```python
from build123d import *

# Parameters (mm, degrees)
ESTRUSIONE_ESTRUSIONE1_DEPTH                         = 4
ESTRUSIONE_ESTRUSIONE2_START                         = -36
ESTRUSIONE_ESTRUSIONE2_DEPTH                         = 36
ESTRUSIONE_ESTRUSIONE3_START                         = -46
ESTRUSIONE_ESTRUSIONE3_DEPTH                         = 46
SMUSSO3_SIZE                                         = 8.0941
SMUSSO3_SIZE2                                        = 11.999996735
SMUSSO2_SIZE                                         = 8.0941
SMUSSO2_SIZE_2                                       = 11.999996735
FORO_LAMATO_PER_VITE_M4_A_TESTA_CILINDRI_D           = 4.5
FORO_LAMATO_PER_VITE_M4_A_TESTA_CILINDRI_DEPTH       = 50
FORO_LAMATO_PER_VITE_M4_A_TESTA_CILINDRI_CBORE_D     = 8
FORO_LAMATO_PER_VITE_M4_A_TESTA_CILINDRI_CBORE_DEPTH = 35.6
FORO_LAMATO_PER_VITE_M4_A_TESTA_CILINDRI_TIP         = 1.351936393
FORO_PER_VITE_M4_1_D                                 = 4.5
FORO_PER_VITE_M4_1_DEPTH                             = 50
FORO_PER_VITE_M4_1_TIP                               = 1.351936393


with BuildPart() as part:
    # Schizzo1 → Estrusione-Estrusione1 (new body)
    with BuildSketch(Plane.XY):
        Polygon((35, 30), (23, 30), (23, 18), (23, 0), (-23, 0), (-23, 18), (-23, 30), (-35, 30), (-35, -12), (35, -12), align=None)
        with BuildLine():
            ThreePointArc((-8, 18), (0, 10), (8, 18))
            Line((8, 18), (23, 18))
            Line((23, 18), (23, 0))
            Line((23, 0), (-23, 0))
            Line((-23, 0), (-23, 18))
            Line((-23, 18), (-8, 18))
        make_face()
    extrude(amount=ESTRUSIONE_ESTRUSIONE1_DEPTH)

    # Schizzo1<3> → Estrusione-Estrusione2 (add)
    with BuildSketch(Plane.XY.offset(ESTRUSIONE_ESTRUSIONE2_START)):
        with BuildLine():
            ThreePointArc((-8, 18), (0, 10), (8, 18))
            Line((8, 18), (23, 18))
            Line((23, 18), (23, 0))
            Line((23, 0), (-23, 0))
            Line((-23, 0), (-23, 18))
            Line((-23, 18), (-8, 18))
        make_face()
    extrude(amount=ESTRUSIONE_ESTRUSIONE2_DEPTH)

    # Schizzo6 → Estrusione-Estrusione3 (add)
    with BuildSketch(Plane(origin=(23, 0, 0), x_dir=(0, 0, -1), z_dir=(1, 0, 0)).offset(ESTRUSIONE_ESTRUSIONE3_START)):
        Polygon((0, 0), (25, 0), (0, -12), align=None)
    extrude(amount=ESTRUSIONE_ESTRUSIONE3_DEPTH)

    # Smusso3
    smusso3_edges = [part.edges().sort_by_distance(p)[0] for p in [
        (-23, 3, 0),
    ]]
    smusso3_side = [part.faces().sort_by_distance(p)[0] for p in [
        (-23, 6.556390977, -16.182957393),
    ]]
    chamfer(smusso3_edges, length=SMUSSO3_SIZE, length2=SMUSSO3_SIZE2, reference=smusso3_side[0])

    # Smusso2
    # the kernel refuses this chamfer: 11.999996735, 8.0941 mm, written as the material it adds along each edge
    with BuildSketch(Plane(origin=(23, -43.002099643, 0), x_dir=(-0.047532142988028575, 0, -0.9988697089125115), z_dir=(0, 1, 0))) as smusso2_piece_1_section:
        Polygon((SMUSSO2_SIZE * 0.998869708913, -SMUSSO2_SIZE * 0.047532142988), (-SMUSSO2_SIZE_2 * 0.047532142989, -SMUSSO2_SIZE_2 * 0.998869708932), (0, 0), align=None)
    smusso2_piece_1 = extrude(amount=61.002099643, mode=Mode.PRIVATE)
    smusso2_piece_1 = split(smusso2_piece_1, bisect_by=Plane(origin=(27.04511503, -8.043833676, -8.242013176), z_dir=(0, 0.9015230574682735, 0.4327310675847713)), keep=Keep.TOP, mode=Mode.PRIVATE)
    add(smusso2_piece_1)

    # Foro lamato per Vite M4 a testa cilindrica piana-1
    with Locations(Plane(origin=(0, 0, -36), x_dir=(-1, 0, 0), z_dir=(0, 0, -1))):
        with Locations((-29, -6), (28.999998368, -6)):
            CounterBoreHole(FORO_LAMATO_PER_VITE_M4_A_TESTA_CILINDRI_D / 2, FORO_LAMATO_PER_VITE_M4_A_TESTA_CILINDRI_CBORE_D / 2, FORO_LAMATO_PER_VITE_M4_A_TESTA_CILINDRI_CBORE_DEPTH, depth=FORO_LAMATO_PER_VITE_M4_A_TESTA_CILINDRI_DEPTH)
            with Locations((0, 0, -(FORO_LAMATO_PER_VITE_M4_A_TESTA_CILINDRI_DEPTH + FORO_LAMATO_PER_VITE_M4_A_TESTA_CILINDRI_TIP / 2))):  # 118° drill point
                Cone(0, FORO_LAMATO_PER_VITE_M4_A_TESTA_CILINDRI_D / 2, FORO_LAMATO_PER_VITE_M4_A_TESTA_CILINDRI_TIP, mode=Mode.SUBTRACT)

    # Foro per Vite M4-1
    with Locations(Plane(origin=(29, 24, 0), x_dir=(-1, 0, 0), z_dir=(0, 0, -1))):
        with Locations((0, 0), (58, 0)):
            Hole(FORO_PER_VITE_M4_1_D / 2, depth=FORO_PER_VITE_M4_1_DEPTH)
            with Locations((0, 0, -(FORO_PER_VITE_M4_1_DEPTH + FORO_PER_VITE_M4_1_TIP / 2))):  # 118° drill point
                Cone(0, FORO_PER_VITE_M4_1_D / 2, FORO_PER_VITE_M4_1_TIP, mode=Mode.SUBTRACT)


solid = part.part
```
Geometry check sheet. Reference: the model listing, model coordinates, mm. A direction names the side the tool comes from. Coordinates: 2 decimals unless noted, no trailing zeros. Order: outer loops, then holes, each group sorted by start corner. A loop starts at its lowest first (then second) coordinate and runs counter-clockwise, first axis right, second up. Notation, with made-up numbers: (39, 26.5) - (87, 26.5) arc R24 cw to (87, 48.5) - close; hole circle Ø8 at (58, 34). An arc over 180 degrees is marked (long way). Answer in a Markdown table with one row per item. Add a question column.
1. Material ranges on L1, parallel to Y at x = 29, z = 2.5; L2, parallel to X at y = -0.5, z = -20; L3, parallel to X at y = -6, z = -3, recorded low to high. Write a range as [from, to].
2. Section check B-B (y = 19). Enter the section's corners in (x, z), plus the area to 3 significant figures.
3. Section check C-C (z = -15). Enter the section's corners in (x, y).
4. Gauge pin test, flat ends, axial feed: pin 1 Ø8 at (x, z) = (-16.5, -25.5) entering from +Y; pin 2 Ø8 at (y, z) = (-5.5, -23) entering from -X; pin 3 Ø8 at (y, z) = (-0.5, -18.5) entering from -X; pin 4 Ø7 at (x, y) = (29, -6) entering from -Z. Record the tip position at first contact, or that the pin passes through.
5. Draft check along X on faces 1 (the face through (0, 9, -36)), 2 (the face through (28.92, 6.12, -4.1)), 3 (the face through (23, 24, 2)), 4 (the face through (-23, 24, 2)). Enter one of: +X half, -X half, draft (parallel to the pull), parting line (faces both ways), or undercut.
6. Access from +Z, -Z, +X, -X, +Y, -Y to the whole of each face (thin tool, end or side, straight path). Record for faces 5 (the face through (23, 8, -22)), 6 (the face through (29, 21.5, 0)), 7 (the face through (0, 0, -31)), 8 (the face through (-23, 8, -22)).
7. Section check A-A (y = 24). Enter the section's corners in (x, z).
Data:
| question | item | result |
|---|---|---|
| 1 | L1 | y = [-12, -8.25], [-3.75, 21.75], [26.25, 30] |
| 1 | L2 | x = [-23, 23] |
| 1 | L3 | x = [-25, 25] |
| 2 | outline | (-35, 0) - (-23, 0) - (-23, 4) - (-35, 4) - close; (23, 0) - (35, 0) - (35, 4) - (23, 4) - close |
| 2 | area | 96.0 mm² |
| 3 | outline | (-23, -4.8) - (23, -4.8) - (23, 18) - (8, 18) arc R8 cw to (-8, 18) - (-23, 18) - close |
| 4 | pin 1 | stops at y = 18 |
| 4 | pin 2 | passes through |
| 4 | pin 3 | stops at x = -23 |
| 4 | pin 4 | stops at z = -0.4 |
| 5 | face 1 | draft |
| 5 | face 2 | +X half |
| 5 | face 3 | undercut |
| 5 | face 4 | undercut |
| 6 | face 5 | -Z, +X, +Y, -Y |
| 6 | face 6 | -Z, +X, -X, +Y |
| 6 | face 7 | -Z, +X, -X, -Y |
| 6 | face 8 | -Z, -X, +Y, -Y |
| 7 | outline | (-35, 0) - (-31.25, 0) - (-31.25, 4) - (-35, 4) - close; (-26.75, 0) - (-23, 0) - (-23, 4) - (-26.75, 4) - close; (23, 0) - (26.75, 0) - (26.75, 4) - (23, 4) - close; (31.25, 0) - (35, 0) - (35, 4) - (31.25, 4) - close |
